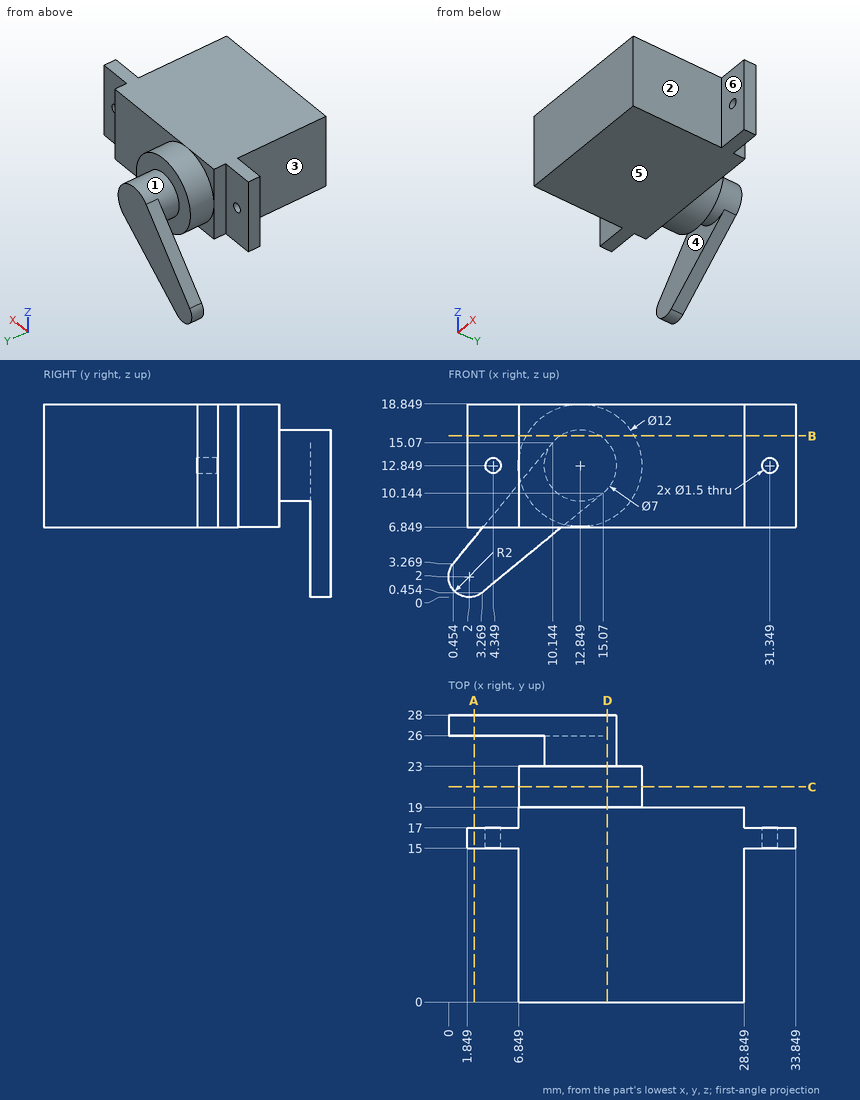
Geometry: see drawing. Coordinates: mm, zero at the bounding-box minimum. A direction names the side the tool comes from. Coordinates: 2 decimals unless noted, no trailing zeros. Order: outer loops, then holes, each group sorted by start corner. A loop starts at its lowest first (then second) coordinate and runs counter-clockwise, first axis right, second up. Notation, with made-up numbers: M -34,56 L -2,56 A16 ccw -2,83 Z; hole C 78.5,-1 d4. An arc over 180 degrees is marked long. Write item = value, one per line. Start each with the question number.
(1) Section B-B on z = 15.75. Output: boundary loops of the cut face in (x, y).
(2) Section D-D on x = 15.5. Output: boundary loops of the cut face in (y, z), and give its area (3 significant figures).
(3) First-contact query: P1, Ø9.5, axis at y = 6, z = 11, coming from the -X side; P2, Ø5, axis at x = 6, z = 15.5, coming from the +Y side; P3, Ø1.5, axis at x = 32, z = 10.5, coming from the +Y side; P4, Ø2, axis at y = 23.5, z = 4.5, coming from the +X side. Flat tips, straight axial feed; report the tip coordinate or a pass-through.
(4) Section C-C on y = 21. Output: boundary loops of the cut face in (x, z), and give its area (3 significant figures).
(5) Section A-A on x = 2.5. Output: boundary loops of the cut face in (y, z).
(6) Pull-direction query (Y, two-part tool) for the marked faces 4, 5 and 6; classes: released by +Y, released by -Y, zero draft, split by the parting line, or undercut.
(7) Line query: line 1 along Y through (x, z) = (2.5, 11.5); line 2 along Y through (x, z) = (22.5, 18); line 3 along Y through (x, z) = (8, 10). Output: solid intervals per line, ascending. Write a range as [from, to].
(8) Reachability of the marked faces 1, 2 and 3 from +Z, -Z, +X, -X, +Y, -Y: full face, straight path, thin tool, end or side. Return the list, or none.
Result set:
q1.outline = M 1.85,15 L 6.85,15 L 6.85,0 L 28.85,0 L 28.85,15 L 33.85,15 L 33.85,17 L 28.85,17 L 28.85,19 L 18.1,19 L 18.1,23 L 14.81,23 L 14.81,28 L 10.89,28 L 10.89,23 L 7.6,23 L 7.6,19 L 6.85,19 L 6.85,17 L 1.85,17 Z
q2.outline = M 0,6.85 L 19,6.85 L 19,7.47 L 23,7.47 L 23,10.56 L 28,10.56 L 28,15.13 L 23,15.13 L 23,18.23 L 19,18.23 L 19,18.85 L 0,18.85 Z
q2.area = 294 mm²
q3.P1 = 6.85
q3.P2 = 23
q3.P3 = 17
q3.P4 = through
q4.outline = C 12.85,12.85 d12
q4.area = 113 mm²
q5.outline = M 15,6.85 L 17,6.85 L 17,18.85 L 15,18.85 Z; M 26,0.06 L 28,0.06 L 28,5.76 L 26,5.76 Z
q6.face_4 = undercut
q6.face_5 = zero draft
q6.face_6 = released by -Y
q7.line_1 = [15, 17]
q7.line_2 = [0, 19]
q7.line_3 = [0, 23], [26, 28]
q8.face_1 = none
q8.face_2 = +Z, -Z, +X, -Y
q8.face_3 = +Z, -Z, -X, -Y
